from build123d import *

# Parameters (mm, degrees)
F0_R     = 5
F1_DEPTH = 15
F0_R_2   = 12
F2_DEPTH = 30


with BuildPart() as f1:
    # F0 (on Top) → F1 (new body)
    with BuildSketch(Plane.XY):
        with BuildLine():
            ThreePointArc((5, 19.364917), (15.811388, 12.247449), (20, 0))
            ThreePointArc((20, 0), (15.811388, -12.247449), (5, -19.364917))
            Line((5, -19.364917), (42.5, -9.682458))
            ThreePointArc((42.5, -9.682458), (50, 0), (42.5, 9.682458))
            Line((42.5, 9.682458), (5, 19.364917))
        make_face()
        with Locations((40, 0)):
            Circle(F0_R, mode=Mode.SUBTRACT)
    extrude(amount=-F1_DEPTH)

    # F0 (on Top) → F2 (join)
    with BuildSketch(Plane.XY):
        with BuildLine():
            ThreePointArc((5, -19.364917), (15.811388, -12.247449), (20, 0))
            ThreePointArc((20, 0), (15.811388, 12.247449), (5, 19.364917))
            ThreePointArc((5, 19.364917), (-20, 0), (5, -19.364917))
        make_face()
        Circle(F0_R_2, mode=Mode.SUBTRACT)
    extrude(amount=-F2_DEPTH)


solid = f1.part
Verification items for the finished model (mm, model axes). Give positions to 0.01 mm unless a question says otherwise; leave off trailing zeros. Write each loop counter-clockwise with the first axis right and the second up, starting at its lowest first coordinate (ties: lowest second). Pieces come first, ordered by that corner, then holes. Notation, with made-up numbers: M 23.5,-17 L 34.5,-17 A15 ccw 34.5,-8 Z; hole C -38,-19 d1. An arc over 180 degrees is marked long. Use CSV: the item, a comma, the result in double quotes.
1) Cross-section at A-A (x = 0). Enter the section's corners in (y, z), plus the area to 3 significant figures.
Final values:
outline,"M -20,-30 L -12,-30 L -12,0 L -20,0 Z; M 12,-30 L 20,-30 L 20,0 L 12,0 Z"
area,"480 mm²"
2) Go/stop test with flat-tipped pins: pin 1 Ø11.5 at (x, y) = (28.5, -7) entering from -Z; pin 2 Ø4 at (x, y) = (9.5, 2.5) entering from -Z; pin 3 Ø10 at (x, z) = (8, -26) entering from -Y; pin 4 Ø6 at (y, z) = (13.5, -19) entering from +X. Record where each tip stops, or that it passes through.
Final values:
pin 1,"z = -15"
pin 2,"through"
pin 3,"y = -19.77"
pin 4,"x = 17.02"
3) Cross-section at D-D (z = -24.75). Enter the section's corners in (x, y), plus the area to 3 significant figures.
Final values:
outline,"M 5,-19.36 A20 ccw 5,19.36 A20 ccw long Z; hole C 0,0 d24"
area,"804 mm²"
4) Cross-section at B-B (z = -14.25). Enter the section's corners in (x, y), plus the area to 3 significant figures.
Final values:
outline,"M 5,-19.36 L 42.5,-9.68 A10 ccw 42.5,9.68 L 5,19.36 A20 ccw long Z; hole C 0,0 d24; hole C 40,0 d10"
area,"1,490 mm²"
5) Release check for a two-part mould opening along X. For faces 1 (the face through (23.49, -14.59, -7.4)), 2 (the face through (15, 0, 0)), 3 (the face through (35, 0, -7)), 4 (the face through (-11.99, 0.53, -14.79)) record: released by +X, released by -X, zero draft, split by the parting line, or undercut.
Final values:
face 1,"released by +X"
face 2,"zero draft"
face 3,"undercut"
face 4,"undercut"
6) Cross-section at C-C (y = 6). Enter the section's corners in (x, z).
Final values:
outline,"M -19.08,-30 L -10.39,-30 L -10.39,0 L -19.08,0 Z; M 10.39,-30 L 19.08,-30 L 19.08,-15 L 48,-15 L 48,0 L 10.39,0 Z"
7) Material ranges on line 1 along X through (y, z) = (-3.5, -8.5); line 2 along Y through (x, z) = (0, -19); line 3 along X through (y, z) = (-7, -2.5) (3 decimals), recorded low to high.
Final values:
line 1,"-19.69 to -11.48, 11.48 to 36.43, 43.57 to 49.37"
line 2,"-20 to -12, 12 to 20"
line 3,"-18.735 to -9.747, 9.747 to 47.141"
